Job drawing, mm, ordinate dimensions from the low corner. One solid piece. A direction names the side the tool comes from. Give positions to 0.01 mm unless a question says otherwise; leave off trailing zeros. Order: outer loops, then holes, each group sorted by start corner. A loop starts at its lowest first (then second) coordinate and runs counter-clockwise, first axis right, second up.
1. Which spindle directions (+Z, -Z, +X, -X, +Y, -Y) get a long thin tool onto all of the face, cutting with end or side? Do the marked faces 4 and 5. Say none if no direction does.
2. Slice it at D-D on y = 16. List the corners of the cut face in (x, z).
3. Slice it at C-C on x = 21.5. List the corners of the cut face in (y, z), and give its area (3 significant figures).
4. Slice it at B-B on x = 18. List the corners of the cut face in (y, z).
5. Probe line 1 (X direction, y = 1.6, z = 3); line 2 (Y direction, x = 17.5, z = 5.5); line 3 (Z direction, x = 18.5, y = 2). List the from-to ranges inside material, lowest first.
6. Mould opens along Z. For the marked faces 1, 2 and 3 say: +Z half, -Z half, draft (parallel to the pull), parting line (faces both ways), or undercut.
7. Drop flat-ended pins along their axis: pin 1 Ø4.5 at (x, z) = (18.5, 3.5) entering from +Y; pin 2 Ø2.5 at (y, z) = (1, 14.5) entering from +X; pin 3 Ø2 at (y, z) = (8, 12) entering from -X. Give the stop position or say it passes through.
8. Slice it at A-A on y = 2.5. List the corners of the cut face in (x, z).
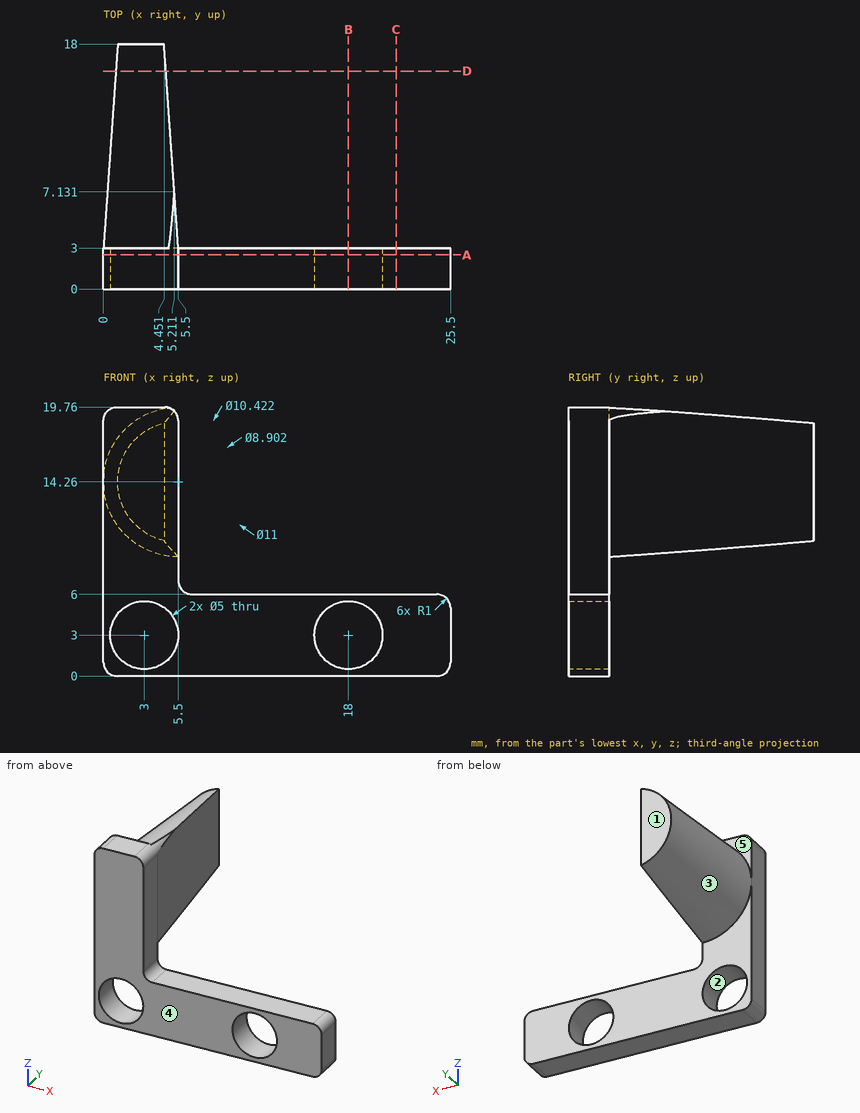
Data:
1. face 4: +Z, -Z, +X, -X, -Y
1. face 5: +Z, -X, +Y
2. outline: (4.59, 9.76) - (4.59, 18.76) arc R4.59 ccw to start
3. outline: (0, 0) - (3, 0) - (3, 6) - (0, 6) - close
3. area: 18.0 mm2
4. outline: (0, 0) - (3, 0) - (3, 0.5) - (0, 0.5) - close; (0, 5.5) - (3, 5.5) - (3, 6) - (0, 6) - close
5. line 1: x = 0 to 0.5, 5.5 to 15.5, 20.5 to 25.5
5. line 2: y = 0 to 3
5. line 3: z = 0 to 0.55, 5.45 to 6
6. face 1: draft
6. face 2: undercut
6. face 3: parting line
7. pin 1: stops at y = 3
7. pin 2: stops at x = 5.5
7. pin 3: stops at x = 0.5
8. outline: (0, 1) arc R1 ccw to (1, 0) - (24.5, 0) arc R1 ccw to (25.5, 1) - (25.5, 5) arc R1 ccw to (24.5, 6) - (6.5, 6) arc R1 cw to (5.5, 7) - (5.5, 18.76) arc R1 ccw to (4.5, 19.76) - (1, 19.76) arc R1 ccw to (0, 18.76) - close; hole circle Ø5 at (3, 3); hole circle Ø5 at (18, 3)
